from build123d import *

# Parameters (mm, degrees)
SKETCH1_W           = 58
SKETCH1_H           = 58
SKETCH1_R           = 2
BOSS_EXTRUDE1_DEPTH = 8
SKETCH13_R          = 15
CUT_EXTRUDE5_DEPTH  = 5
BOSS_EXTRUDE7_DEPTH = 8
SKETCH21_W          = 84
SKETCH21_H          = 10
BOSS_EXTRUDE8_DEPTH = 114
SKETCH22_W          = 9.98
SKETCH22_H          = 9.98
BOSS_EXTRUDE9_DEPTH = 114
SKETCH29_W          = 20
SKETCH29_H          = 6
CUT_EXTRUDE6_DEPTH  = 40
SKETCH30_W          = 10
SKETCH30_H          = 76
CUT_EXTRUDE7_DEPTH  = 138.320792308
SKETCH31_R          = 2.5
CUT_EXTRUDE8_DEPTH  = 4
SKETCH34_R          = 2.5
CUT_EXTRUDE9_DEPTH  = 10
SKETCH36_R          = 2.5
CUT_EXTRUDE10_DEPTH = 20
CUT_EXTRUDE12_DEPTH = 15


with BuildPart() as part:
    # Sketch1 → Boss-Extrude1 (new body)
    with BuildSketch(Plane.XY):
        Rectangle(SKETCH1_W, SKETCH1_H)
        with Locations((0, 24)):
            Circle(SKETCH1_R, mode=Mode.SUBTRACT)
        with Locations((-24, 24)):
            Circle(SKETCH1_R, mode=Mode.SUBTRACT)
        with Locations((24, 0)):
            Circle(SKETCH1_R, mode=Mode.SUBTRACT)
        with Locations((0, -24)):
            Circle(SKETCH1_R, mode=Mode.SUBTRACT)
        with Locations((-24, 0)):
            Circle(SKETCH1_R, mode=Mode.SUBTRACT)
        with Locations(Location((24, -24, 0), (0, 0, 180))):
            Circle(SKETCH1_R, mode=Mode.SUBTRACT)
        with Locations((24, 24)):
            Circle(SKETCH1_R, mode=Mode.SUBTRACT)
        with Locations(Location((-24, -24, 0), (0, 0, 180))):
            Circle(SKETCH1_R, mode=Mode.SUBTRACT)
    extrude(amount=BOSS_EXTRUDE1_DEPTH)

    # Sketch13 → Cut-Extrude5 (cut)
    with BuildSketch(Plane.XY.offset(8)):
        Circle(SKETCH13_R)
    extrude(amount=-CUT_EXTRUDE5_DEPTH, mode=Mode.SUBTRACT)

    # Sketch15 → Boss-Extrude7 (add)
    with BuildSketch(Plane.XY):
        Polygon((29, -29), (-29, -29), (-29, 29), (-42, 29), (-42, -29), (-42, -47), (42, -47), (42, -29), (42, 29), (29, 29), align=None)
    extrude(amount=BOSS_EXTRUDE7_DEPTH)

    # Sketch21 → Boss-Extrude8 (add)
    with BuildSketch(Plane.XY.offset(8)):
        with Locations((0, -42)):
            Rectangle(SKETCH21_W, SKETCH21_H)
    extrude(amount=BOSS_EXTRUDE8_DEPTH)

    # Sketch22 → Boss-Extrude9 (add)
    with BuildSketch(Plane.XY.offset(8)):
        with Locations((-37.01, -32.01)):
            Rectangle(SKETCH22_W, SKETCH22_H)
    extrude(amount=BOSS_EXTRUDE9_DEPTH)

    # Sketch29 → Cut-Extrude6 (cut)
    with BuildSketch(Plane.ZY.offset(42)):
        with Locations((103, -44)):
            Rectangle(SKETCH29_W, SKETCH29_H)
        with Locations((63, -44)):
            Rectangle(SKETCH29_W, SKETCH29_H)
        with Locations((23, -44)):
            Rectangle(SKETCH29_W, SKETCH29_H)
    extrude(amount=-CUT_EXTRUDE6_DEPTH, mode=Mode.SUBTRACT)

    # Sketch30 → Cut-Extrude7 (cut, through all)
    with BuildSketch(Plane.XY.offset(122)):
        with Locations((37, -9)):
            Rectangle(SKETCH30_W, SKETCH30_H)
    extrude(amount=-CUT_EXTRUDE7_DEPTH, mode=Mode.SUBTRACT)

    # Sketch31 → Cut-Extrude8 (cut)
    with BuildSketch(Plane.XZ.offset(41)):
        with Locations(Location((-7, 103, 0), (0, 0, 270))):
            Circle(SKETCH31_R)
        with Locations(Location((-7, 63, 0), (0, 0, 90))):
            Circle(SKETCH31_R)
        with Locations(Location((-7, 23, 0), (0, 0, 270))):
            Circle(SKETCH31_R)
    extrude(amount=-CUT_EXTRUDE8_DEPTH, mode=Mode.SUBTRACT)

    # Sketch34 → Cut-Extrude9 (cut)
    with BuildSketch(Plane.ZY.offset(42)):
        with Locations((43, -33)):
            Circle(SKETCH34_R)
        with Locations((83, -33)):
            Circle(SKETCH34_R)
    extrude(amount=-CUT_EXTRUDE9_DEPTH, mode=Mode.SUBTRACT)

    # Sketch36 → Cut-Extrude10 (cut)
    with BuildSketch(Plane.XZ.offset(41)):
        with Locations(Location((-37, 103, 0), (0, 0, 270))):
            Circle(SKETCH36_R)
        with Locations(Location((-37, 23, 0), (0, 0, 270))):
            Circle(SKETCH36_R)
        with Locations(Location((-37, 63, 0), (0, 0, 270))):
            Circle(SKETCH36_R)
    extrude(amount=-CUT_EXTRUDE10_DEPTH, mode=Mode.SUBTRACT)

    # Sketch37 → Cut-Extrude12 (cut)
    with BuildSketch(Plane.XY.offset(8)):
        Polygon((-42, -27.02), (-32.02, 0), (-32.02, 29), (-42, 29), align=None)
    extrude(amount=-CUT_EXTRUDE12_DEPTH, mode=Mode.SUBTRACT)


solid = part.part
Geometry check sheet. Reference: the model listing, model coordinates, mm. A direction names the side the tool comes from. Give positions to 0.01 mm unless a question says otherwise; leave off trailing zeros. Order: outer loops, then holes, each group sorted by start corner. A loop starts at its lowest first (then second) coordinate and runs counter-clockwise, first axis right, second up. Notation, with made-up numbers: (78, 25) - (113, 25) arc R24 ccw to (113, 54) - close; hole circle Ø9 at (43.25, -38). An arc over 180 degrees is marked (long way). Answer as a JSON object with one key per item and string values.
(1) Material ranges on line 1 (Y direction, x = 24, z = 3); line 2 (Y direction, x = -39.75, z = 43); line 3 (Z direction, x = -27.5, y = -34), recorded low to high.
Report:
{"line 1": "-47 to -26, -22 to -2, 2 to 22, 26 to 29", "line 2": "-47 to -35.5, -30.5 to -27.02", "line 3": "0 to 8"}
(2) Cross-section at B-B (z = 43). Record the cut outline in (x, y).
Report:
{"outline": "(-42, -47) - (32, -47) - (32, -37) - (-32.02, -37) - (-32.02, -35.5) - (-42, -35.5) - close; (-42, -30.5) - (-32.02, -30.5) - (-32.02, -27.02) - (-42, -27.02) - close"}
(3) Cross-section at A-A (x = 24). Record the cut outline in (y, z).
Report:
{"outline": "(-47, 0) - (-26, 0) - (-26, 8) - (-37, 8) - (-37, 122) - (-47, 122) - close; (-22, 0) - (-2, 0) - (-2, 8) - (-22, 8) - close; (2, 0) - (22, 0) - (22, 8) - (2, 8) - close; (26, 0) - (29, 0) - (29, 8) - (26, 8) - close"}
(4) Draft check along Y on faces 1 (the cylindrical face through (-6.249, -39.028, 100.615)), 2 (the flat face through (-40, -27.02, 64)), 3 (the cylindrical face through (-14.985, 0.66, 5.535)). Enter one of: released by +Y, released by -Y, zero draft, split by the parting line, or undercut.
Report:
{"face 1": "zero draft", "face 2": "released by +Y", "face 3": "undercut"}
(5) Tool access check on faces 4 (the flat face through (-14, -11, 8)), 5 (the flat face through (-2, -44, 103)), 6 (the flat face through (-32.02, 14, 4)). Record the directions out of +Z, -Z, +X, -X, +Y, -Y that give a thin tool (end or side, any length) a straight path to the whole face; none if there is none.
Report:
{"face 4": "+Z, +X, +Y", "face 5": "-X, -Y", "face 6": "+Z, -Z, -X, +Y"}
(6) Cross-section at D-D (z = 63). Record the cut outline in (x, y).
Report:
{"outline": "(-42, -41) - (-39.5, -41) - (-39.5, -27.02) - (-42, -27.02) - close; (-34.5, -41) - (-9.5, -41) - (-9.5, -37) - (-32.02, -37) - (-32.02, -27.02) - (-34.5, -27.02) - close; (-4.5, -41) - (-2, -41) - (-2, -47) - (32, -47) - (32, -37) - (-4.5, -37) - close"}
(7) Cross-section at C-C (y = -33). Record the cut outline in (x, z), then the cut area to 3 significant figures.
Report:
{"outline": "(-42, 0) - (32, 0) - (32, 8) - (-32.02, 8) - (-32.02, 40.5) - (-42, 40.5) - close; (-42, 45.5) - (-32.02, 45.5) - (-32.02, 80.5) - (-42, 80.5) - close; (-42, 85.5) - (-32.02, 85.5) - (-32.02, 122) - (-42, 122) - close; hole circle Ø5 at (-37, 23); hole circle Ø5 at (-37, 63); hole circle Ø5 at (-37, 103)", "area": "1,570 mm^2"}
(8) Depth check by flat-ended pin: pin 1 Ø6.5 at (x, y) = (-18, -43) entering from -Z; pin 2 Ø3 at (x, y) = (24, -24) entering from -Z; pin 3 Ø10 at (x, z) = (8.5, 79.5) entering from +Y; pin 4 Ø16 at (x, z) = (-28, 24.5) entering from -Y. Enter the tip coordinate at first touch or a pass-through.
Report:
{"pin 1": "z = 0", "pin 2": "through", "pin 3": "y = -37", "pin 4": "y = -41"}
